The drawing under review shows one solid part. Ordinate dimensions are in mm from its lowest x, y, z. A direction names the side the tool comes from. Round coordinates to 2 decimals unless told otherwise and drop trailing zeros. Write each loop counter-clockwise with the first axis right and the second up, starting at its lowest first coordinate (ties: lowest second). Pieces come first, ordered by that corner, then holes.
Item 1: Machinability: for the marked faces 1 and 2, which of the approach directions +Z, -Z, +X, -X, +Y, -Y give a long, thin tool a straight path to every point of the face, cutting with its end or side? Answer none if there is none.
Item 2: Clearance check with flat-ended pins moving along their axes: pin 1 Ø2 at (x, y) = (30.5, 84) entering from +Z; pin 2 Ø11.5 at (x, z) = (35.5, 24) entering from +Y. State where each tip first meets the part, or that it passes through.
Item 3: Add section A-A (x = 12). Give the boundary of the cut face in (y, z), plus the area to 3 significant figures.
Item 4: Add section B-B (z = 28.5). Give the boundary of the cut face in (x, y), plus the area to 3 significant figures.
Item 5: To check wall thickness, follow L1, parallel to Y at x = 22.5, z = 32.5. State the ranges of the line that lie inside material, in increasing order.
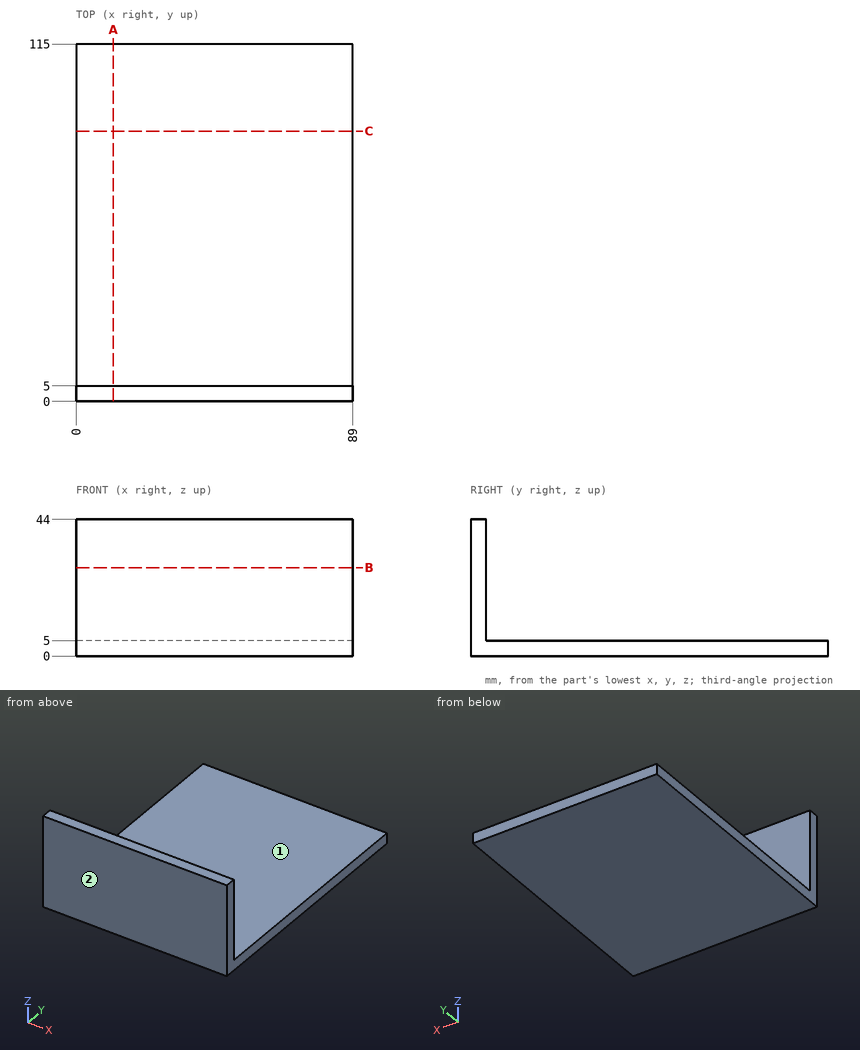
Numbers:
1. face 1: +Z, +X, -X, +Y
1. face 2: +Z, -Z, +X, -X, -Y
2. pin 1: stops at z = 5
2. pin 2: stops at y = 5
3. outline: (0, 0) - (115, 0) - (115, 5) - (5, 5) - (5, 44) - (0, 44) - close
3. area: 770 mm2
4. outline: (0, 0) - (89, 0) - (89, 5) - (0, 5) - close
4. area: 445 mm2
5. L1: y = 0 to 5
